```python
from build123d import *

# Parameters (mm, degrees)
F2_W      = 60
F2_H      = 8
F2_R      = 3
F4_DEPTH  = 4
F5_R      = 3.99999
F6_R      = 10
F7_DEPTH  = 3
F3_R      = 1.3
F8_DEPTH  = 4.001
F9_W      = 25
F9_H      = 8
F10_DEPTH = 1
F11_DEPTH = 2


# Not quite as in the source:
# - a fillet or chamfer is up to 0.001 mm smaller than in the source, because OpenCascade refuses the exact size


with BuildPart() as f4:
    # F2 (on face) → F4 (new body)
    with BuildSketch(Plane.XY):
        with Locations((0, 38)):
            Rectangle(F2_W, F2_H)
        with Locations((-26, 38)):
            Circle(F2_R, mode=Mode.SUBTRACT)
        Polygon((1.1402667816, 36.025), (0, 36.025), (-1.1402667816, 36.025), (-2.2805335633, 38), (-1.1402667816, 39.975), (0, 39.975), (1.1402667816, 39.975), (2.2805335633, 38), align=None, mode=Mode.SUBTRACT)
        with Locations((26, 38)):
            Circle(F2_R, mode=Mode.SUBTRACT)
        Polygon((-1.1402667816, 36.025), (0, 36.025), (1.1402667816, 36.025), (2.2805335633, 38), (1.1402667816, 39.975), (0, 39.975), (-1.1402667816, 39.975), (-2.2805335633, 38), align=None)
        with Locations((-26, 38)):
            Circle(F2_R)
        with Locations((26, 38)):
            Circle(F2_R)
    extrude(amount=F4_DEPTH)

    # F5 (radius 4 in the source; OpenCascade refuses exactly that, so slightly less here)
    f5_edges = [f4.edges().sort_by_distance(p)[0] for p in [
        (-30, 42, 2),
        (-30, 34, 2),
        (30, 42, 2),
        (30, 34, 2),
    ]]
    fillet(f5_edges, radius=F5_R)

    # F6 (on face) → F7 (join)
    with BuildSketch(Plane.XY.offset(4)):
        with Locations((0, 38)):
            Circle(F6_R)
    extrude(amount=-F7_DEPTH)

    # F3 (on face) → F8 (cut, through all)
    with BuildSketch(Plane.XY):
        with Locations((0, 38)):
            Circle(F3_R)
    extrude(amount=F8_DEPTH, mode=Mode.SUBTRACT)

    # F9 (on face) → F10 (cut)
    with BuildSketch(Plane.XY):
        with Locations((17.5, 38)):
            Rectangle(F9_W, F9_H)
        with Locations((-17.5, 38)):
            Rectangle(F9_W, F9_H)
    extrude(amount=F10_DEPTH, mode=Mode.SUBTRACT)

    # F2 (on face) → F11 (cut)
    with BuildSketch(Plane.XY):
        Polygon((-1.1402667816, 36.025), (0, 36.025), (1.1402667816, 36.025), (2.2805335633, 38), (1.1402667816, 39.975), (0, 39.975), (-1.1402667816, 39.975), (-2.2805335633, 38), align=None)
    extrude(amount=F11_DEPTH, mode=Mode.SUBTRACT)


solid = f4.part
```
Here's how the part is built. I have some questions about the finished solid (model axes, mm). A direction names the side the tool comes from. Round coordinates to 2 decimals unless told otherwise and drop trailing zeros. Loops run counter-clockwise (first coordinate to the right, second up) from the corner with the lowest first, then second, coordinate; pieces in that order, holes last.
1. For faces 5 (the face through (0, 39.975, 1)), 6 (the face through (-18, 42, 2)), 7 (the face through (-5, 37.9, 0.5)), which set-ups out of +Z, -Z, +X, -X, +Y, -Y let a thin tool reach every point of the face, with its end or its side?
Answers:
face 5: -Z
face 6: +Z, -Z, -X, +Y
face 7: -Z, -X, +Y, -Y
2. Suppose I cut it at D-D, the plane x = -23. Please give me the cut outline in (y, z), and give its area (3 significant figures).
Answers:
outline: (34, 1) - (42, 1) - (42, 4) - (34, 4) - close
area: 24.0 mm2
3. Will these pins go through, and if not, where does the flat tip stop? pin 1 (0.6 mm diameter, centred on x = 0, z = 0.5, fed in from +Y); pin 2 (3 mm diameter, centred on x = 1, y = 37, fed in from -Z); pin 3 (8 mm diameter, centred on x = -15, y = 43.5, fed in from -Z); pin 4 (0.6 mm diameter, centred on x = -0.5, z = 0.5, fed in from -Y).
Answers:
pin 1: stops at y = 42
pin 2: stops at z = 0
pin 3: stops at z = 1
pin 4: stops at y = 34
4. Thinking about a two-plate mould opening in Y: for faces 1 (the face through (-2, 37, 0)), 2 (the face through (-0.1, 34, 0.5)), 3 (the face through (-1.72, 37.03, 0.99)), 4 (the face through (17, 42, 2)), which applies, released by +Y, released by -Y, zero draft, split by the parting line, or undercut?
Answers:
face 1: zero draft
face 2: released by -Y
face 3: undercut
face 4: released by +Y
5. Suppose I cut it at C-C, the plane y = 35. Please give me the cut outline in (x, z).
Answers:
outline: (-28.65, 1) - (-5, 1) - (-5, 0) - (5, 0) - (5, 1) - (28.65, 1) - (28.65, 4) - (-28.65, 4) - close
6. If I drill on probe 1 along X at (y, z) = (38, 2.9); probe 2 along Z at (x, y) = (-14, 34.25); probe 3 along Y at (x, z) = (14, 2.4), over which ranges is the centre line in solid material (lowest first)?
Answers:
probe 1: x = -30 to -1.3, 1.3 to 30
probe 2: z = 1 to 4
probe 3: y = 34 to 42
7. Suppose I cut it at B-B, the plane x = 0. Please give me the cut outline in (y, z) (3 decimals), and give its area (3 significant figures).
Answers:
outline: (28, 1) - (34, 1) - (34, 0) - (36.025, 0) - (36.025, 2) - (36.7, 2) - (36.7, 4) - (28, 4) - close; (39.3, 2) - (39.975, 2) - (39.975, 0) - (42, 0) - (42, 1) - (48, 1) - (48, 4) - (39.3, 4) - close
area: 54.9 mm2
